Here's how the part is built. I have some questions about the finished solid (model axes, mm). A direction names the side the tool comes from. Give positions to 0.01 mm unless a question says otherwise; leave off trailing zeros. Write each loop counter-clockwise with the first axis right and the second up, starting at its lowest first coordinate (ties: lowest second). Pieces come first, ordered by that corner, then holes. Notation, with made-up numbers: (52.5, 29.25) - (79.5, 29.25) arc R22 ccw to (79.5, 47.25) - close; hole circle Ø7 at (-25.5, -12). An arc over 180 degrees is marked (long way). Use a Markdown table: item, result.
```python
from build123d import *

# Parameters (mm, degrees)
CROQUIS1_W                = 15
CROQUIS1_H                = 15
SALIENTE_EXTRUIR1_DEPTH   = 30
SALIENTE_EXTRUIR1_2_DEPTH = 30
CROQUIS2_R                = 5.5
CORTAR_EXTRUIR1_DEPTH     = 30
CROQUIS3_R                = 5
CORTAR_EXTRUIR2_DEPTH     = 30
CROQUIS5_W                = 115
CROQUIS5_H                = 60
SALIENTE_EXTRUIR3_DEPTH   = 5
CROQUIS6_W                = 54.898151636
CROQUIS6_H                = 43
SALIENTE_EXTRUIR4_DEPTH   = 4.7625
CROQUIS7_R                = 2
CORTAR_EXTRUIR3_DEPTH     = 4.7625
CROQUIS8_R                = 6
CORTAR_EXTRUIR4_DEPTH     = 10
CROQUIS9_W                = 40
CROQUIS9_H                = 6.3
SALIENTE_EXTRUIR5_DEPTH   = 35
REDONDEO1_R               = 10
CORTAR_EXTRUIR5_REACH     = 95.087
CROQUIS10_R               = 4
REDONDEO3_R               = 1
REDONDEO4_R               = 1
REDONDEO5_R               = 1
REDONDEO6_R               = 1
REDONDEO8_R               = 1
CHAFL_N1_SIZE             = 1


with BuildPart() as part:
    # Croquis1 → Saliente-Extruir1 (new body)
    with BuildSketch(Plane(origin=(0, 0, 0), x_dir=(1, 0, 0), z_dir=(0, 1, 0))):
        with Locations((-37.5, 20.000000005)):
            Rectangle(CROQUIS1_W, CROQUIS1_H)
    extrude(amount=SALIENTE_EXTRUIR1_DEPTH)

    # Croquis2 → Cortar-Extruir1 (cut)
    with BuildSketch(Plane(origin=(0, 0, -27.500000005), x_dir=(-1, 0, 0), z_dir=(0, 0, -1))):
        with Locations((37.5, 22.231754591)):
            Circle(CROQUIS2_R)
    extrude(amount=-CORTAR_EXTRUIR1_DEPTH, mode=Mode.SUBTRACT)



with BuildPart() as body_2:
    # Croquis1 → Saliente-Extruir1 2 (new body)
    with BuildSketch(Plane(origin=(0, 0, 0), x_dir=(1, 0, 0), z_dir=(0, 1, 0))):
        with Locations((42.5, 20.000000005)):
            Rectangle(CROQUIS1_W, CROQUIS1_H)
    extrude(amount=SALIENTE_EXTRUIR1_2_DEPTH)

    # Croquis3 → Cortar-Extruir2 (cut)
    with BuildSketch(Plane(origin=(0, 0, -27.500000005), x_dir=(-1, 0, 0), z_dir=(0, 0, -1))):
        with Locations((-42.5, 22.231754591)):
            Circle(CROQUIS3_R)
    extrude(amount=-CORTAR_EXTRUIR2_DEPTH, mode=Mode.SUBTRACT)


with BuildPart() as part_1:
    add(part.part)

    add(body_2.part)  # Saliente-Extruir3 merges body 2
    # Croquis5 → Saliente-Extruir3 (add)
    with BuildSketch(Plane(origin=(0, 0, 0), x_dir=(1, 0, 0), z_dir=(0, 1, 0))):
        with Locations((3.699250586, 15.919051757)):
            Rectangle(CROQUIS5_W, CROQUIS5_H)
    extrude(amount=-SALIENTE_EXTRUIR3_DEPTH)

    # Croquis6 → Saliente-Extruir4 (add)
    with BuildSketch(Plane.XY.offset(14.080948243)):
        with Locations((2.330070819, 16.5)):
            Rectangle(CROQUIS6_W, CROQUIS6_H)
    extrude(amount=SALIENTE_EXTRUIR4_DEPTH)

    # Croquis7 → Cortar-Extruir3 (cut)
    with BuildSketch(Plane.XY.offset(18.843448243)):
        with Locations((17.730070819, 22.23)):
            Circle(CROQUIS7_R)
        with Locations((10.071882042, 8.965627944)):
            Circle(CROQUIS7_R)
        with Locations((-5.244495512, 8.965627944)):
            Circle(CROQUIS7_R)
        with Locations((-12.902684289, 22.23)):
            Circle(CROQUIS7_R)
        with Locations((-5.244495512, 35.494372056)):
            Circle(CROQUIS7_R)
        with Locations((10.071882042, 35.494372056)):
            Circle(CROQUIS7_R)
    extrude(amount=-CORTAR_EXTRUIR3_DEPTH, mode=Mode.SUBTRACT)

    # Croquis8 → Cortar-Extruir4 (cut)
    with BuildSketch(Plane.XY.offset(18.843448243)):
        with Locations((2.5, 22.231754591)):
            Circle(CROQUIS8_R)
    extrude(amount=-CORTAR_EXTRUIR4_DEPTH, mode=Mode.SUBTRACT)

    # Croquis9 → Saliente-Extruir5 (add)
    with BuildSketch(Plane(origin=(0, -5, 0), x_dir=(-1, 0, 0), z_dir=(0, -1, 0))):
        with Locations((-2.600505063, 33.750505063)):
            Rectangle(CROQUIS9_W, CROQUIS9_H)
        with Locations((-2.600505063, -8.549494937)):
            Rectangle(CROQUIS9_W, CROQUIS9_H)
    extrude(amount=SALIENTE_EXTRUIR5_DEPTH)

    # Redondeo1
    redondeo1_edges = [part_1.edges().sort_by_distance(p)[0] for p in [
        (22.600505063, -40, 8.549494937),
        (-17.399494937, -40, 8.549494937),
        (-17.399494937, -40, -33.750505063),
        (22.600505063, -40, -33.750505063),
    ]]
    fillet(redondeo1_edges, radius=REDONDEO1_R)

    # Cortar-Extruir5: up to this face of the body (flat: up to its plane)
    cortar_extruir5_end = Plane(part_1.part.faces().sort_by_distance((2.600505063, -22.017171968, -36.900505063))[0])
    # Croquis10 → Cortar-Extruir5 (cut, up to the picked face)
    with BuildSketch(Plane.XY.offset(11.699494937), mode=Mode.PRIVATE) as cortar_extruir5_sk1:
        with Locations((2.600505063, -30)):
            Circle(CROQUIS10_R)
    cortar_extruir5_tool1 = split(extrude(cortar_extruir5_sk1.sketch, amount=-CORTAR_EXTRUIR5_REACH, mode=Mode.PRIVATE), bisect_by=cortar_extruir5_end, keep=Keep.BOTH, mode=Mode.PRIVATE)
    add(cortar_extruir5_tool1.solids().sort_by(Axis((2.600505, -30, 11.699495), (0, 0, -1)))[0], mode=Mode.SUBTRACT)

    # Redondeo3
    redondeo3_edges = [part_1.edges().sort_by_distance(p)[0] for p in [
        (2.600505063, -40, -36.900505063),
        (2.600505063, -40, -30.600505063),
        (-17.399494937, -17.5, -30.600505063),
        (22.600505063, -17.5, -30.600505063),
        (-14.470562748, -37.071067812, -30.600505063),
        (19.671572875, -37.071067812, -30.600505063),
        (22.600505063, -17.5, -36.900505063),
        (-17.399494937, -17.5, -36.900505063),
        (-14.470562748, -37.071067812, -36.900505063),
        (19.671572875, -37.071067812, -36.900505063),
        (2.600505063, -40, 11.699494937),
        (2.600505063, -40, 5.399494937),
        (-17.399494937, -17.5, 11.699494937),
        (22.600505063, -17.5, 11.699494937),
        (-14.470562748, -37.071067812, 11.699494937),
        (19.671572875, -37.071067812, 11.699494937),
        (22.600505063, -17.5, 5.399494937),
        (-17.399494937, -17.5, 5.399494937),
        (-14.470562748, -37.071067812, 5.399494937),
        (19.671572875, -37.071067812, 5.399494937),
    ]]
    fillet(redondeo3_edges, radius=REDONDEO3_R)

    # Redondeo4
    redondeo4_edges = [part_1.edges().sort_by_distance(p)[0] for p in [
        (61.199250586, -2.5, 14.080948243),
        (-53.800749414, -2.5, 14.080948243),
        (-53.800749414, -2.5, -45.919051757),
        (61.199250586, -2.5, -45.919051757),
    ]]
    fillet(redondeo4_edges, radius=REDONDEO4_R)

    # Redondeo5
    redondeo5_edges = [part_1.edges().sort_by_distance(p)[0] for p in [
        (-30, 30, -20.000000005),
        (35, 30, -20.000000005),
        (50, 30, -20.000000005),
        (-45, 30, -20.000000005),
    ]]
    fillet(redondeo5_edges, radius=REDONDEO5_R)

    # Redondeo6
    redondeo6_edges = [part_1.edges().sort_by_distance(p)[0] for p in [
        (-25.119004999, 38, 16.462198243),
        (29.779146637, 38, 16.462198243),
    ]]
    fillet(redondeo6_edges, radius=REDONDEO6_R)

    # Redondeo8
    redondeo8_edges = [part_1.edges().sort_by_distance(p)[0] for p in [
        (2.330070819, -5, 18.843448243),
    ]]
    fillet(redondeo8_edges, radius=REDONDEO8_R)

    # Chaflán1
    chafl_n1_edges = [part_1.edges().sort_by_distance(p)[0] for p in [
        (-38.959877207, 0, 14.080948243),
        (61.199250586, 0, -15.919051757),
        (3.699250586, 0, -45.919051757),
        (-53.800749414, 0, -15.919051757),
        (60.906357367, 0, -45.626158538),
        (-53.507856195, 0, -45.626158538),
        (-53.507856195, 0, 13.788055024),
        (60.906357367, 0, 13.788055024),
        (61.199250586, -5, -15.919051757),
        (-38.959877207, -5, 14.080948243),
        (-53.800749414, -5, -15.919051757),
        (3.699250586, -5, -45.919051757),
        (60.906357367, -5, -45.626158538),
        (-53.507856195, -5, -45.626158538),
        (-53.507856195, -5, 13.788055024),
        (60.906357367, -5, 13.788055024),
        (44.989198611, 0, 14.080948243),
        (44.989198611, -5, 14.080948243),
    ]]
    chamfer(chafl_n1_edges, length=CHAFL_N1_SIZE)


solid = part_1.part
```
Item 1: Thinking about a two-plate mould opening in Z: for faces 6 (the flat face through (3, -22, -30.601)), 7 (the cylindrical face through (-33.4, 25.9, -20.1)), 8 (the flat face through (2, 13, 18.843)), 9 (the flat face through (3, -22, -36.901)), which applies, +Z half, -Z half, draft (parallel to the pull), parting line (faces both ways), or undercut?
Values:
| item | result |
|---|---|
| face 6 | undercut |
| face 7 | draft |
| face 8 | +Z half |
| face 9 | -Z half |
Item 2: For faces 1 (the flat face through (-39, -2, 14.081)), 2 (the flat face through (22.601, -17, 9)), 3 (the flat face through (50, 14, -20)), 4 (the flat face through (-38, 11, -12.5)), 5 (the flat face through (-17.399, -17, 9)), which set-ups out of +Z, -Z, +X, -X, +Y, -Y let a thin tool reach every point of the face, with its end or its side?
Values:
| item | result |
|---|---|
| face 1 | +Z, -X, +Y, -Y |
| face 2 | +Z, -Z, +X, -Y |
| face 3 | +Z, -Z, +X, +Y |
| face 4 | +Z, +X, -X, +Y |
| face 5 | +Z, -Z, -X, -Y |
Item 3: If we section it at C-C, the plane x = 24.5: Write out the boundary of the cut face in (y, z).
Values:
| item | result |
|---|---|
| outline | (-5, -44.92) - (-4, -45.92) - (-1, -45.92) - (0, -44.92) - (0, 14.08) - (38, 14.08) - (38, 18.84) - (-4, 18.84) arc R1 ccw to (-5, 17.84) - close |
Item 4: If we section it at D-D, the plane z = -18: Write out the boundary of the cut face in (x, y), plus the area to 3 significant figures.
Values:
| item | result |
|---|---|
| outline | (-53.8, -4) - (-52.8, -5) - (60.2, -5) - (61.2, -4) - (61.2, -1) - (60.2, 0) - (50, 0) - (50, 29) arc R1 ccw to (49, 30) - (36, 30) arc R1 ccw to (35, 29) - (35, 0) - (-30, 0) - (-30, 29) arc R1 ccw to (-31, 30) - (-44, 30) arc R1 ccw to (-45, 29) - (-45, 0) - (-52.8, 0) - (-53.8, -1) - close; hole circle Ø11 at (-37.5, 22.23); hole circle Ø10 at (42.5, 22.23) |
| area | 1,300 mm2 |
Item 5: If we section it at B-B, the plane y = -18.5: Write out the boundary of the cut face in (x, z).
Values:
| item | result |
|---|---|
| outline | (-17.4, -35.9) arc R1 ccw to (-16.4, -36.9) - (21.6, -36.9) arc R1 ccw to (22.6, -35.9) - (22.6, -31.6) arc R1 ccw to (21.6, -30.6) - (-16.4, -30.6) arc R1 ccw to (-17.4, -31.6) - close; (-17.4, 6.4) arc R1 ccw to (-16.4, 5.4) - (21.6, 5.4) arc R1 ccw to (22.6, 6.4) - (22.6, 10.7) arc R1 ccw to (21.6, 11.7) - (-16.4, 11.7) arc R1 ccw to (-17.4, 10.7) - close |
Item 6: Will these pins go through, and if not, where does the flat tip stop? pin 1 Ø3.5 at (x, y) = (-5.24, 8.97) entering from -Z; pin 2 Ø11.5 at (x, y) = (2, 15.5) entering from -Z; pin 3 Ø4 at (x, z) = (-35, 5) entering from -Y; pin 4 Ø4 at (y, z) = (-16.5, -29) entering from +X.
Values:
| item | result |
|---|---|
| pin 1 | passes through |
| pin 2 | stops at z = 14.08 |
| pin 3 | stops at y = -5 |
| pin 4 | stops at x = 22.4 |
Item 7: I need wall thicknesses on line 1 along X through (y, z) = (22, 15); line 2 along Y through (x, z) = (42.5, -16.75); line 3 along Y through (x, z) = (-9, -1). Which ranges of each line are inside material? Lowest first, please. Write a range as [from, to].
Values:
| item | result |
|---|---|
| line 1 | x = [-25.12, -14.89], [-10.92, -3.5], [8.5, 15.74], [19.72, 29.78] |
| line 2 | y = [-5, 17.23], [27.23, 30] |
| line 3 | y = [-5, 0] |
Item 8: If we section it at A-A, the plane x = -37.5: Write out the boundary of the cut face in (y, z), plus the area to 3 significant figures.
Values:
| item | result |
|---|---|
| outline | (-5, -44.92) - (-4, -45.92) - (-1, -45.92) - (0, -44.92) - (0, -27.5) - (16.73, -27.5) - (16.73, -12.5) - (0, -12.5) - (0, 13.08) - (-1, 14.08) - (-4, 14.08) - (-5, 13.08) - close; (27.73, -27.5) - (30, -27.5) - (30, -12.5) - (27.73, -12.5) - close |
| area | 583 mm2 |
